Work out the finished part from the listing and answer in its coordinate system (mm). Face numbers are marked on the shaded views. A direction names the side the tool comes from. Round coordinates to 2 decimals unless told otherwise and drop trailing zeros. Loops run counter-clockwise (first coordinate to the right, second up) from the corner with the lowest first, then second, coordinate; pieces in that order, holes last. Notation, with made-up numbers: (51, 88) - (69, 88) arc R27 cw to (69, 104) - close; hole circle Ø8 at (-28, 12). An arc over 180 degrees is marked (long way). Answer as CSV lines item,"result". Start each with the question number.
Q1. Section C-C on y = -14.5 is taken. Write down the section's boundary in (x, z).
Q2. The mould has two halves that part along X. Classify the marked faces 1, 2, 3 and 4: +X half, -X half, draft (parallel to the pull), parting line (faces both ways), or undercut.
Q3. Section A-A on x = 0 is taken. Write down the section's boundary in (y, z), then the cut area to 4 significant figures.
Q4. Section D-D on z = -6 is taken. Write down the section's boundary in (x, y).
Q5. Each of these flat-tipped pins is pushed along its axis until it touches: pin 1 Ø3 at (x, y) = (-42.5, 17.6) entering from -Z; pin 2 Ø1.2 at (x, y) = (-0.5, 9.5) entering from +Z; pin 3 Ø5 at (y, z) = (11, 11.5) entering from +X. Where does it stop, or does it pass through?
Q6. Straight lines are drawn through the part: L1, parallel to Z at x = -34, y = 25.5; L2, parallel to X at y = 25.5, z = 13.5; L3, parallel to Z at x = 28, y = 8. For each, find the intervals that lie inside material, in ascending order. Write a range as [from, to].
Q7. For the marked faces 5, 6 and 7, determine the directions among +Z, -Z, +X, -X, +Y, -Y from which every point of the face is accessible in a straight line to the end or side of a thin tool.
Q8. Section B-B on z = 9.5 is taken. Count the separate pieces of the cut face and the enclosed holes in it, then the cut area to 3 significant figures.
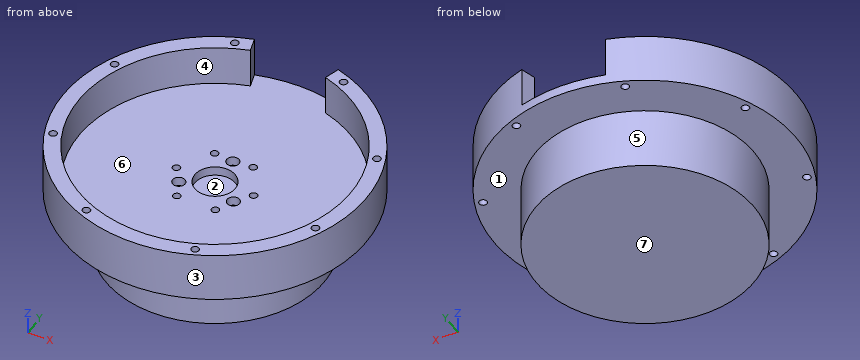
Autodesk Inventor part; units mm, degrees
ref_plane "YZ Plane" through (0, 0, 0) normal (1, 0, 0) x (0, 1, 0)
ref_plane "XZ Plane" through (0, 0, 0) normal (0, 1, 0) x (-1, 0, 0)
ref_plane "XY Plane" through (0, 0, 0) normal (0, 0, 1) x (1, 0, 0)
sketch "スケッチ1" plane through (0, 0, 0) normal (0, 0, 1) x (1, 0, 0)
  circle A0 centre (0, 0) radius 48.5
  dimension "d0" = 97
extrude "押し出し1" add sketch "スケッチ1" along normal blind 24
sketch "スケッチ2" plane through (0, 0, 24) normal (0, 0, 1) x (1, 0, 0)
  line L0 (0, 0) -> (-27.4547, 66.2816)
  line L1 (0, 0) -> (26.2443, 63.3594)
  circle A0 centre (0, 0) radius 46
  line L2 (0, 0) -> (0, 57.2216)
  point P0 (-17.6034, 42.4985)
  point P1 (17.6034, 42.4985)
  point P2 (-42.4985, -17.6034)
  point P3 (-42.4985, 17.6034)
  point P4 (17.6034, -42.4985)
  point P5 (-17.6034, -42.4985)
  point P6 (42.4985, 17.6034)
  point P7 (42.4985, -17.6034)
  dimension "d3" = 92
  dimension "d4" = 45
  dimension "d8" = 360
  dimension "d45" = 22.5
hole "穴1" at (-17.6034, 42.4985, 24) at (17.6034, 42.4985, 24) at (-42.4985, -17.6034, 24) at (-42.4985, 17.6034, 24) at (17.6034, -42.4985, 24) at (-17.6034, -42.4985, 24) at (42.4985, 17.6034, 24) at (42.4985, -17.6034, 24) direction (0, 0, -1) diameter 2.459 end through all
sketch "スケッチ3" plane through (0, 0, 0) normal (0, 0, -1) x (-1, 0, 0)
  circle A0 centre (0, 0) radius 12.5
  line L0 (0, 0) -> (-8.9989, 15.5865)
  line L1 (0, 0) -> (0, 21.1985)
  point P0 (-6.25, 10.8253)
  point P1 (-12.5, 0)
  point P2 (-6.25, -10.8253)
  point P3 (6.25, -10.8253)
  point P4 (12.5, 0)
  point P5 (6.25, 10.8253)
  dimension "d17" = 25
  dimension "d18" = 30
  dimension "d21" = 360
hole "穴2" at (6.25, 10.8253, 0) at (12.5, 0, 0) at (6.25, -10.8253, 0) at (-6.25, -10.8253, 0) at (-12.5, 0, 0) at (-6.25, 10.8253, 0) direction (0, 0, 1) diameter 2.459 end through all
sketch "スケッチ4" plane through (0, 0, 0) normal (0, 0, -1) x (-1, 0, 0)
  circle A0 centre (0, 0) radius 10.2
  point P0 (0, 10.2)
  point P1 (0, 10.2)
  point P2 (-8.8335, -5.1)
  point P3 (8.8335, -5.1)
  dimension "d30" = 20.4
  dimension "d33" = 360
hole "穴3" at (0, 10.2, 0) at (8.8335, -5.1, 0) at (-8.8335, -5.1, 0) direction (0, 0, 1) diameter 4 end through all
sketch "スケッチ5" plane through (0, 0, 24) normal (0, 0, 1) x (1, 0, 0)
  circle A0 centre (0, 0) radius 43.5
  dimension "d42" = 87
extrude "押し出し2" cut sketch "スケッチ5" against normal blind 21
sketch "スケッチ6" plane through (0, 0, 24) normal (0, 0, 1) x (1, 0, 0)
  circle A0 centre (0, 0) radius 48.5
  circle A1 centre (0, 0) radius 43.5
  line L0 (-13.5797, 46.5601) -> (0, 0)
  line L1 (0, 0) -> (13.6731, 46.8801)
  circle A2 centre (-17.6034, 42.4985) radius 1.2295
  circle A3 centre (17.6034, 42.4985) radius 1.2295
  arc A4 (13.5797, 46.5601) -> (-13.5797, 46.5601) centre (0, 0) ccw
  arc A5 (12.1798, 41.7601) -> (-12.1798, 41.7601) centre (0, 0) ccw
  dimension "d46" = 5
  dimension "d47" = 5
extrude "押し出し3" cut sketch "スケッチ6" against normal blind 21 contours L1 A1 L0 A0 picked at (-1.3696, 46.624)
sketch "スケッチ7" plane through (0, 0, 0) normal (0, 0, -1) x (-1, 0, 0)
  circle A0 centre (0, 0) radius 6.5
  dimension "d50" = 13
extrude "押し出し4" cut sketch "スケッチ7" against normal blind 10
sketch "スケッチ8" plane through (0, 0, 24) normal (0, 0, 1) x (1, 0, 0)
  circle A0 centre (0, 0) radius 48.5
extrude "押し出し5" cut sketch "スケッチ8" against normal blind 8
sketch "スケッチ9" plane through (0, 0, 0) normal (0, 0, -1) x (-1, 0, 0)
  circle A0 centre (0, 0) radius 35
  dimension "d55" = 70
extrude "押し出し6" add sketch "スケッチ9" along normal blind 20
sketch "スケッチ10" plane through (0, 0, 3) normal (0, 0, 1) x (1, 0, 0)
  point P0 (0, 0)
properties part number "legparts_01(five)"
Findings:
1,outline,"(-46.28, 0) - (-31.86, 0) - (-31.86, -20) - (31.86, -20) - (31.86, 0) - (46.28, 0) - (46.28, 16) - (41.01, 16) - (41.01, 3) - (-41.01, 3) - (-41.01, 16) - (-46.28, 16) - close"
2,face 1,"draft"
2,face 2,"undercut"
2,face 3,"parting line"
2,face 4,"undercut"
3,outline,"(-48.5, 0) - (-35, 0) - (-35, -20) - (35, -20) - (35, 0) - (48.5, 0) - (48.5, 3) - (12.2, 3) - (12.2, 0) - (8.2, 0) - (8.2, 3) - (6.5, 3) - (6.5, 0) - (-6.5, 0) - (-6.5, 3) - (-43.5, 3) - (-43.5, 16) - (-48.5, 16) - close"
3,area,"1,705 mm^2"
4,outline,"circle Ø70 at (0, 0)"
5,pin 1,"stops at z = 0"
5,pin 2,"stops at z = 0"
5,pin 3,"stops at x = 47.75"
6,L1,"z = [0, 3]"
6,L2,"x = [-41.26, -35.24], [35.24, 41.26]"
6,L3,"z = [-20, 3]"
7,face 5,"-Z"
7,face 6,"+Z"
7,face 7,"-Z, +X, -X, +Y, -Y"
8,separate pieces,"1"
8,enclosed holes,"8"
8,area,"1,280 mm^2"
